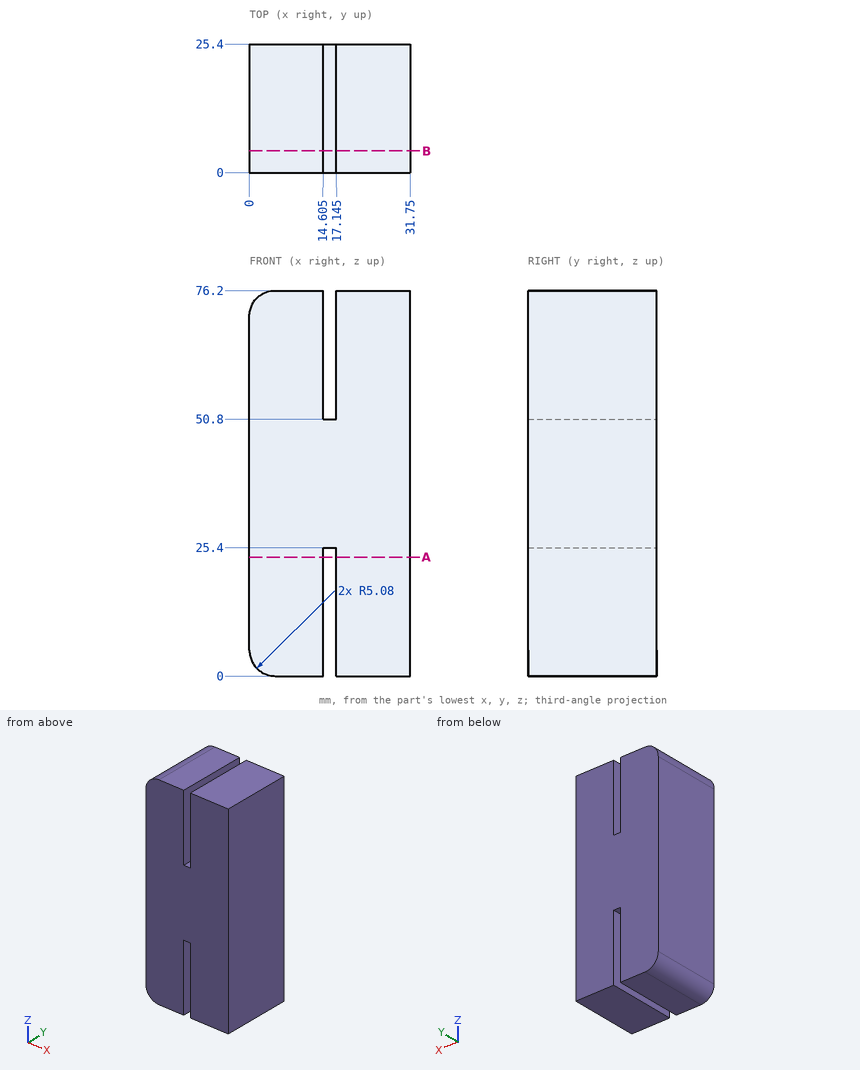
Design review of the part shown in the three views and the two pictorial views. Dimensions are in mm from the part's minimum x, y and z. Round coordinates to 2 decimals unless told otherwise and drop trailing zeros. Loops run counter-clockwise (first coordinate to the right, second up) from the corner with the lowest first, then second, coordinate; pieces in that order, holes last. Notation, with made-up numbers: (-19.5, 38) -> (7.5, 38) arc R35 ccw to (7.5, 77) -> close; hole circle Ø7 at (64, -30). An arc over 180 degrees is marked (long way). Use one line per item in the form item = value. Start each with the question number.
Q1. Wall thickness on line 1 along X through (y, z) = (7.25, 10) (3 decimals); line 2 along Z through (x, y) = (16, 18.5); line 3 along Z through (x, y) = (4, 20.75): over which ranges is each line inside the solid? List them lowest first. Write a range as [from, to].
Q2. We need section A-A on z = 23.5. Give the boundary of the cut face in (x, y) (3 decimals).
Q3. We need section B-B on y = 4.25. Give the boundary of the cut face in (x, z) (3 decimals).
Q4. For pin 1 Ø0.8 at (x, y) = (16.5, 15.5) entering from +Z, flat-tipped, find the tip position at first contact; note if it passes through.
Calculated:
q1.line_1 = [0, 14.605], [17.145, 31.75]
q1.line_2 = [25.4, 50.8]
q1.line_3 = [0.12, 76.08]
q2.outline = (0, 0) -> (14.605, 0) -> (14.605, 25.4) -> (0, 25.4) -> close; (17.145, 0) -> (31.75, 0) -> (31.75, 25.4) -> (17.145, 25.4) -> close
q3.outline = (0, 5.08) arc R5.08 ccw to (5.08, 0) -> (14.605, 0) -> (14.605, 25.4) -> (17.145, 25.4) -> (17.145, 0) -> (31.75, 0) -> (31.75, 76.2) -> (17.145, 76.2) -> (17.145, 50.8) -> (14.605, 50.8) -> (14.605, 76.2) -> (5.08, 76.2) arc R5.08 ccw to (0, 71.12) -> close
q4.pin_1 = 50.8
